Could you check a few things on this model? Use its own coordinates, in mm. Face numbers are marked on the shaded views. Give positions to 0.01 mm unless a question says otherwise; leave off trailing zeros. Order: outer loops, then holes, each group sorted by start corner. A loop starts at its lowest first (then second) coordinate and runs counter-clockwise, first axis right, second up. Notation, with made-up numbers: (6.5, 75) - (23.5, 75) arc R25 ccw to (23.5, 111) - close; hole circle Ø7 at (-18.5, 54). An arc over 180 degrees is marked (long way). One line per question, with ' | ' between items. Start each with the question number.
1. Imagine slicing it at A-A (z = -9). Please give me the cut outline in (x, y), and give its area (3 significant figures).
2. Imagine slicing it at B-B (x = 3.25). Please give me the cut outline in (y, z).
3. I need wall thicknesses on probe 1 along X at (y, z) = (-1, -9.5); probe 2 along Y at (x, z) = (2.75, -7); probe 3 along X at (y, z) = (-4.5, -8). Which ranges of each line are inside material? Lowest first, please. Write a range as from..to.
4. If we mould it in two halves opening along X, with no side actions, what happens to the marked faces 1, 2 and 3? For each: released by +X, released by -X, zero draft, split by the parting line, or undercut.
```python
from build123d import *

# Parameters (mm, degrees)
BOSS_EXTRUDE1_DEPTH = 45
CHAMFER1_SIZE       = 1


with BuildPart() as part:
    # Sketch1 → Boss-Extrude1 (new body)
    with BuildSketch(Plane.XY):
        Polygon((6, -5), (13.25, -5), (13.25, 5), (-13.25, 5), (-13.25, -5), (-6, -5), (-6, 0), (6, 0), align=None)
    extrude(amount=-BOSS_EXTRUDE1_DEPTH)

    # Chamfer1
    chamfer1_edges = [part.edges().sort_by_distance(p)[0] for p in [
        (-13.25, -5, -22.5),
        (-13.25, 5, -22.5),
        (13.25, 5, -22.5),
        (13.25, -5, -22.5),
    ]]
    chamfer(chamfer1_edges, length=CHAMFER1_SIZE)


solid = part.part
```
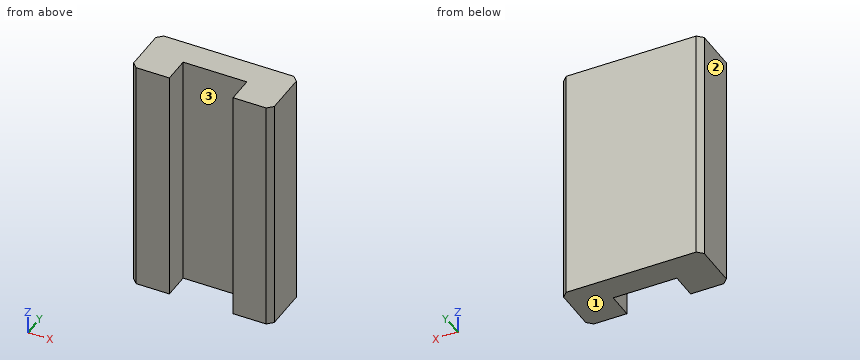
Results found:
1) outline: (-13.25, -4) - (-12.25, -5) - (-6, -5) - (-6, 0) - (6, 0) - (6, -5) - (12.25, -5) - (13.25, -4) - (13.25, 4) - (12.25, 5) - (-12.25, 5) - (-13.25, 4) - close | area: 203 mm2
2) outline: (0, -45) - (5, -45) - (5, 0) - (0, 0) - close
3) probe 1: x = -13.25..-6, 6..13.25 | probe 2: y = 0..5 | probe 3: x = -12.75..-6, 6..12.75
4) face 1: zero draft | face 2: released by -X | face 3: undercut
